The model under review builds one solid part; all positions refer to its coordinate system, in mm. Give positions to 0.01 mm unless a question says otherwise; leave off trailing zeros. Loops run counter-clockwise (first coordinate to the right, second up) from the corner with the lowest first, then second, coordinate; pieces in that order, holes last. Notation, with made-up numbers: (4.5, 11.25) -> (47.5, 11.25) arc R37 cw to (47.5, 47.25) -> close; hole circle Ø3 at (-10.5, -14). An arc over 180 degrees is marked (long way). Write each question's results on one line, items separated by ' | '. Start each with the question number.
Q1. We need section A-A (z = 0). Write out the cut boundary in (x, y).
Q2. We need section B-B (x = 2.75). Write out the cut boundary in (y, z), plus the area to 3 significant figures.
Q3. Wall thickness on L1, parallel to X at y = -1.25, z = 0.2; L2, parallel to Y at x = 1.75, z = -0.05; L3, parallel to Y at x = 0.75, z = -0.2: over which ranges is each line inside the solid? List them lowest first. Write a range as [from, to].
Q4. Insertion check: pin 1 Ø2 at (x, y) = (5.5, 2.5) entering from +Z. The pin has a flat end and moves straight along its axis. Give the tip position at first contact, or say it passes through.
Q5. We need section C-C (y = 1.5). Write out the cut boundary in (x, z).
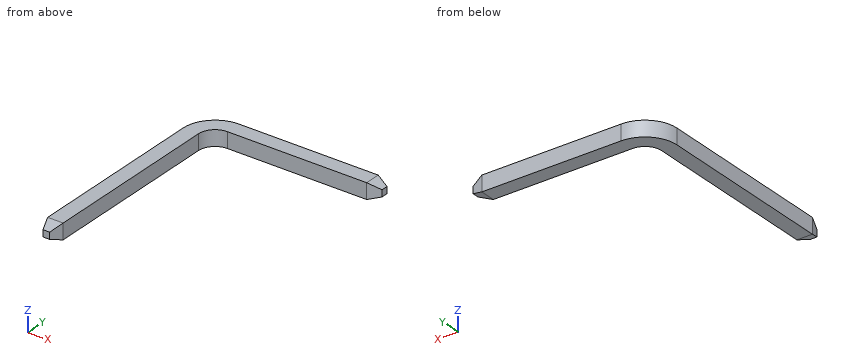
from build123d import *
from OCP.BRepFilletAPI import BRepFilletAPI_MakeChamfer

# Parameters (mm, degrees)
SKETCH_1_W      = 0.64
SKETCH_1_H      = 0.64
CHAMFER_1_SIZE  = 0.5
CHAMFER_1_SIZE2 = 0.181985117
CHAMFER_2_SIZE  = 0.5
CHAMFER_2_SIZE2 = 0.181985117


with BuildPart() as part:
    # По траектории1: sweep along a path in Эскиз2
    with BuildLine(Plane.XY) as sweep_1_path:
        Line((7.25, 4.75), (1, 4.75))
        ThreePointArc((1, 4.75), (0.292893219, 4.457106781), (0, 3.75))
        Line((0, 3.75), (0, 0))
        Line((0, 0), (0, -4.25))
    # Эскиз1 → По траектории1 (sweep)
    with BuildSketch(Plane(origin=(0, 0, 0), x_dir=(1, 0, 0), z_dir=(0, 1, 0))):
        Rectangle(SKETCH_1_W, SKETCH_1_H)
    sweep(path=sweep_1_path.line)

    # Фаска1: one chamfer whose edges measure the first distance from different faces: ONE call of the kernel's chamfer builder (chamfer() names one face for all edges)
    chamfer_1_edges_1 = [part.edges().sort_by_distance(p)[0] for p in [
        (7.25, 5.07, 0),
    ]]
    chamfer_1_side_1 = [part.faces().sort_by_distance(p)[0] for p in [
        (4.125, 5.07, 0),
    ]]
    chamfer_1_edges_2 = [part.edges().sort_by_distance(p)[0] for p in [
        (7.25, 4.75, 0.32),
    ]]
    chamfer_1_side_2 = [part.faces().sort_by_distance(p)[0] for p in [
        (4.125, 4.949930312, 0.32),
    ]]
    chamfer_1_edges_3 = [part.edges().sort_by_distance(p)[0] for p in [
        (7.25, 4.43, 0),
    ]]
    chamfer_1_side_3 = [part.faces().sort_by_distance(p)[0] for p in [
        (4.125, 4.43, 0),
    ]]
    chamfer_1_edges_4 = [part.edges().sort_by_distance(p)[0] for p in [
        (7.25, 4.75, -0.32),
    ]]
    chamfer_1_side_4 = [part.faces().sort_by_distance(p)[0] for p in [
        (4.125, 4.550069688, -0.32),
    ]]
    chamfer_1 = BRepFilletAPI_MakeChamfer(part.part.solid().wrapped)
    for e in chamfer_1_edges_1:
        chamfer_1.Add(CHAMFER_1_SIZE, CHAMFER_1_SIZE2, e.wrapped, chamfer_1_side_1[0].wrapped)  # the first distance lies on this face
    for e in chamfer_1_edges_2:
        chamfer_1.Add(CHAMFER_1_SIZE, CHAMFER_1_SIZE2, e.wrapped, chamfer_1_side_2[0].wrapped)  # the first distance lies on this face
    for e in chamfer_1_edges_3:
        chamfer_1.Add(CHAMFER_1_SIZE, CHAMFER_1_SIZE2, e.wrapped, chamfer_1_side_3[0].wrapped)  # the first distance lies on this face
    for e in chamfer_1_edges_4:
        chamfer_1.Add(CHAMFER_1_SIZE, CHAMFER_1_SIZE2, e.wrapped, chamfer_1_side_4[0].wrapped)  # the first distance lies on this face
    add(Compound.cast(chamfer_1.Shape()), mode=Mode.REPLACE)

    # Фаска2: one chamfer whose edges measure the first distance from different faces: ONE call of the kernel's chamfer builder (chamfer() names one face for all edges)
    chamfer_2_edges_1 = [part.edges().sort_by_distance(p)[0] for p in [
        (0, -4.25, 0.32),
    ]]
    chamfer_2_side_1 = [part.faces().sort_by_distance(p)[0] for p in [
        (3.875, 4.953018249, 0.32),
    ]]
    chamfer_2_edges_2 = [part.edges().sort_by_distance(p)[0] for p in [
        (0.32, -4.25, 0),
    ]]
    chamfer_2_side_2 = [part.faces().sort_by_distance(p)[0] for p in [
        (0.32, -0.25, 0),
    ]]
    chamfer_2_edges_3 = [part.edges().sort_by_distance(p)[0] for p in [
        (0, -4.25, -0.32),
    ]]
    chamfer_2_side_3 = [part.faces().sort_by_distance(p)[0] for p in [
        (3.875, 4.546981751, -0.32),
    ]]
    chamfer_2_edges_4 = [part.edges().sort_by_distance(p)[0] for p in [
        (-0.32, -4.25, 0),
    ]]
    chamfer_2_side_4 = [part.faces().sort_by_distance(p)[0] for p in [
        (-0.32, -0.25, 0),
    ]]
    chamfer_2 = BRepFilletAPI_MakeChamfer(part.part.solid().wrapped)
    for e in chamfer_2_edges_1:
        chamfer_2.Add(CHAMFER_2_SIZE, CHAMFER_2_SIZE2, e.wrapped, chamfer_2_side_1[0].wrapped)  # the first distance lies on this face
    for e in chamfer_2_edges_2:
        chamfer_2.Add(CHAMFER_2_SIZE, CHAMFER_2_SIZE2, e.wrapped, chamfer_2_side_2[0].wrapped)  # the first distance lies on this face
    for e in chamfer_2_edges_3:
        chamfer_2.Add(CHAMFER_2_SIZE, CHAMFER_2_SIZE2, e.wrapped, chamfer_2_side_3[0].wrapped)  # the first distance lies on this face
    for e in chamfer_2_edges_4:
        chamfer_2.Add(CHAMFER_2_SIZE, CHAMFER_2_SIZE2, e.wrapped, chamfer_2_side_4[0].wrapped)  # the first distance lies on this face
    add(Compound.cast(chamfer_2.Shape()), mode=Mode.REPLACE)


solid = part.part
Output:
1) outline: (-0.32, -3.75) -> (-0.14, -4.25) -> (0.14, -4.25) -> (0.32, -3.75) -> (0.32, 3.75) arc R0.68 cw to (1, 4.43) -> (6.75, 4.43) -> (7.25, 4.61) -> (7.25, 4.89) -> (6.75, 5.07) -> (1, 5.07) arc R1.32 ccw to (-0.32, 3.75) -> close
2) outline: (4.43, -0.32) -> (5.07, -0.32) -> (5.07, 0.32) -> (4.43, 0.32) -> close | area: 0.410 mm2
3) L1: [-0.32, 0.32] | L2: [4.43, 5.07] | L3: [4.38, 5.05]
4) pin 1: through
5) outline: (-0.32, -0.32) -> (0.32, -0.32) -> (0.32, 0.32) -> (-0.32, 0.32) -> close
